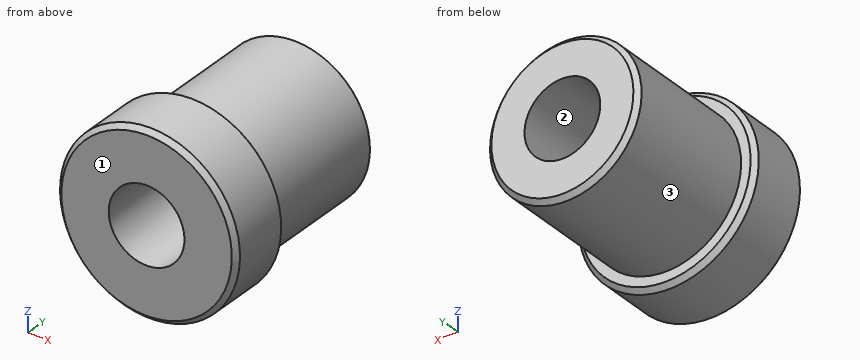
from build123d import *

# Parameters (mm, degrees)
SKETCH1_R           = 9.5
BOSS_EXTRUDE1_DEPTH = 7
SKETCH2_R           = 8
BOSS_EXTRUDE2_DEPTH = 15
SKETCH3_R           = 4
CUT_EXTRUDE1_DEPTH  = 26.777897509
CHAMFER1_SIZE       = 0.5


with BuildPart() as part:
    # Sketch1 → Boss-Extrude1 (new body)
    with BuildSketch(Plane(origin=(0, 0, 0), x_dir=(1, 0, 0), z_dir=(0, 1, 0))):
        with Locations(Location((0, 0, 0), (0, 0, 270))):
            Circle(SKETCH1_R)
    extrude(amount=BOSS_EXTRUDE1_DEPTH)

    # Sketch2 → Boss-Extrude2 (add)
    with BuildSketch(Plane(origin=(0, 7, 0), x_dir=(1, 0, 0), z_dir=(0, 1, 0))):
        with Locations(Location((0, 0, 0), (0, 0, 270))):
            Circle(SKETCH2_R)
    extrude(amount=BOSS_EXTRUDE2_DEPTH)

    # Sketch3 → Cut-Extrude1 (cut, through all)
    with BuildSketch(Plane(origin=(0, 22, 0), x_dir=(1, 0, 0), z_dir=(0, 1, 0))):
        with Locations(Location((0, 0, 0), (0, 0, 270))):
            Circle(SKETCH3_R)
    extrude(amount=-CUT_EXTRUDE1_DEPTH, mode=Mode.SUBTRACT)

    # Chamfer1
    chamfer1_edges = [part.edges().sort_by_distance(p)[0] for p in [
        (0, 0, -9.5),
        (0, 7, -9.5),
        (0, 22, -8),
    ]]
    chamfer(chamfer1_edges, length=CHAMFER1_SIZE)


solid = part.part
The model under review builds one solid part; all positions refer to its coordinate system, in mm. Face numbers are marked on the shaded views. Give positions to 0.01 mm unless a question says otherwise; leave off trailing zeros. Write each loop counter-clockwise with the first axis right and the second up, starting at its lowest first coordinate (ties: lowest second). Pieces come first, ordered by that corner, then holes. Notation, with made-up numbers: M 51,5.25 L 108,5.25 A36 ccw 108,41.25 Z; hole C -12.5,-34 d2. An arc over 180 degrees is marked long. One line per question, with ' | ' between items. Start each with the question number.
Item 1: We need section C-C on y = 3.5. Write out the cut boundary in (x, z), plus the area to 3 significant figures.
Item 2: For pin 1 (2 mm diameter, centred on x = -7, y = 4.5, fed in from -Z); pin 2 (5 mm diameter, centred on x = 6, y = 5, fed in from -Z); pin 3 (6 mm diameter, centred on y = 9, z = -6, fed in from -X), all flat-tipped, find the tip position at first contact; note any pin that passes through.
Item 3: We need section B-B on z = 0. Write out the cut boundary in (x, y), plus the area to 3 significant figures.
Item 4: We need section D-D on y = 19.75. Write out the cut boundary in (x, z), plus the area to 3 significant figures.
Item 5: Draft analysis for pull direction Z (two halves, no side actions). For the marked faces 1, 2 and 3, state which applies: released by +Z, released by -Z, zero draft, split by the parting line, or undercut.
Item 6: We need section A-A on x = 0. Write out the cut boundary in (y, z), plus the area to 3 significant figures.
Item 7: Wall thickness on line 1 (X direction, y = 12.75, z = 0); line 2 (Z direction, x = -2, y = 4.5); line 3 (X direction, y = 6.25, z = 0.5): over which ranges is each line inside the solid? List them lowest first. Write a range as from..to.
Results found:
1) outline: C 0,0 d19; hole C 0,0 d8 | area: 233 mm2
2) pin 1: stops at z = -7.37 | pin 2: stops at z = -8.83 | pin 3: stops at x = -8.45
3) outline: M -9.5,0.5 L -9,0 L -4,0 L -4,22 L -7.5,22 L -8,21.5 L -8,7 L -9,7 L -9.5,6.5 Z; M 4,0 L 9,0 L 9.5,0.5 L 9.5,6.5 L 9,7 L 8,7 L 8,21.5 L 7.5,22 L 4,22 Z | area: 196 mm2
4) outline: C 0,0 d16; hole C 0,0 d8 | area: 151 mm2
5) face 1: zero draft | face 2: undercut | face 3: split by the parting line
6) outline: M 0,-9 L 0.5,-9.5 L 6.5,-9.5 L 7,-9 L 7,-8 L 21.5,-8 L 22,-7.5 L 22,-4 L 0,-4 Z; M 0,4 L 22,4 L 22,7.5 L 21.5,8 L 7,8 L 7,9 L 6.5,9.5 L 0.5,9.5 L 0,9 Z | area: 196 mm2
7) line 1: x = -8..-4, 4..8 | line 2: z = -9.29..-3.46, 3.46..9.29 | line 3: x = -9.49..-3.97, 3.97..9.49
